Answer from the drawing. Dimensions are ordinates in mm from the lowest x, y and z of the part. A direction names the side the tool comes from. Give positions to 0.01 mm unless a question says otherwise; leave off trailing zeros. Order: outer loops, then holes, each group sorted by start corner. A loop starts at its lowest first (then second) coordinate and runs counter-clockwise, first axis right, second up. Notation, with made-up numbers: (66, 64.5) - (119, 64.5) arc R16 cw to (119, 79.5) - close; hole circle Ø1 at (89.25, -22.75). An arc over 180 degrees is marked (long way). Use a Markdown table: item, result. Add a question column.
1) Find section D-D, the plane x = 2. Determine the outline of the cut face in (y, z).
2) Flat-ended cylindrical pins translate along their axes: pin 1 (10 mm diameter, centred on x = 2.5, y = 22.5, fed in from -Z); pin 2 (10 mm diameter, centred on x = 6.5, z = 9, fed in from -Y); pin 3 (11.5 mm diameter, centred on x = 10, y = 10, fed in from -Z); pin 4 (2 mm diameter, centred on x = 10.5, y = 8.5, fed in from -Z). Find the tip coordinate at first contact, or state that the pin passes through.
3) Find section A-A, the plane y = 35. Determine the outline of the cut face in (x, z).
4) Straight lines are drawn through the part: line 1 (Y direction, x = 10, z = 2.05); line 2 (Y direction, x = 10, z = 27.1); line 3 (Z direction, x = 6.75, y = 28). For each, find the intervals that lie inside material, in ascending order.
5) The mould has two halves that part along X. Classify the marked faces 4, 5 and 6: released by +X, released by -X, zero draft, split by the parting line, or undercut.
6) Find section B-B, the plane x = 10. Determine the outline of the cut face in (y, z).
7) For the marked faces 1, 2 and 3, determine the directions among +Z, -Z, +X, -X, +Y, -Y from which every point of the face is accessible in a straight line to the end or side of a thin tool.
8) Find section C-C, the plane z = 26.5. Determine the outline of the cut face in (x, y), plus the area to 3 significant figures.
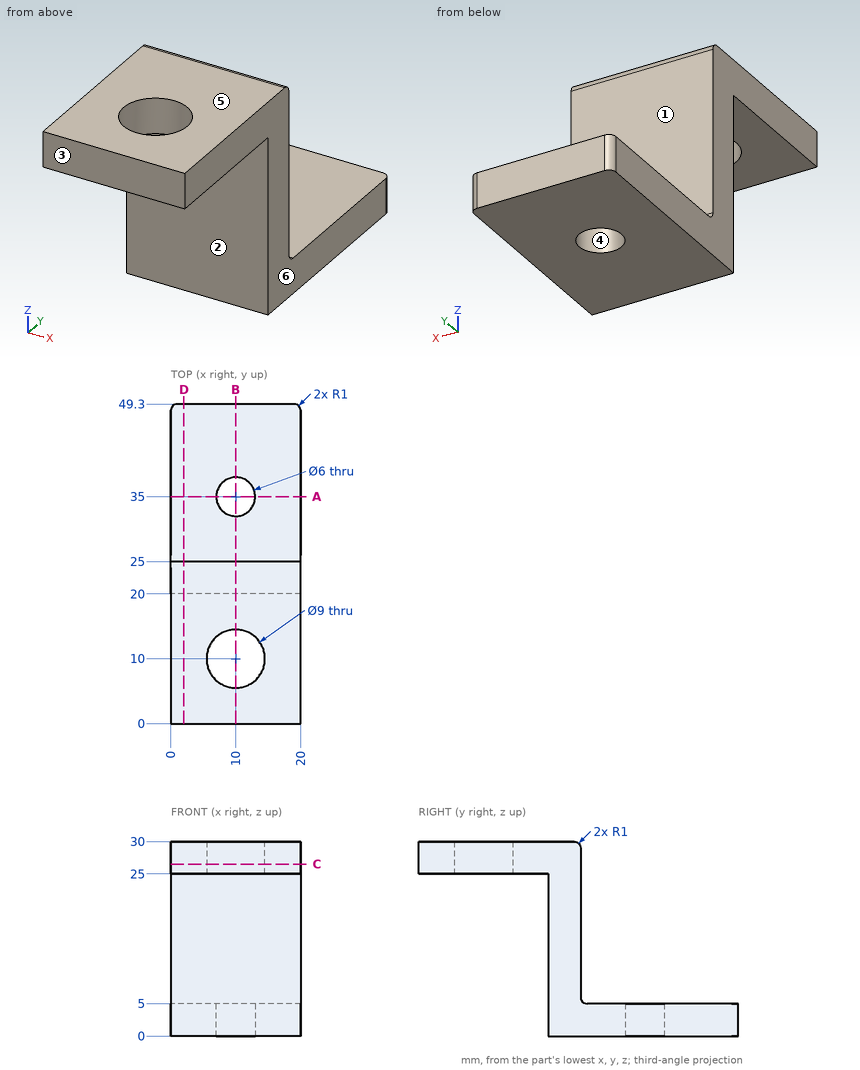
The answers:
| question | item | result |
|---|---|---|
| 1 | outline | (0, 25) - (20, 25) - (20, 0) - (49.3, 0) - (49.3, 5) - (26, 5) arc R1 cw to (25, 6) - (25, 29) arc R1 ccw to (24, 30) - (0, 30) - close |
| 2 | pin 1 | z = 0 |
| 2 | pin 2 | y = 20 |
| 2 | pin 3 | z = 25 |
| 2 | pin 4 | through |
| 3 | outline | (0, 0) - (7, 0) - (7, 5) - (0, 5) - close; (13, 0) - (20, 0) - (20, 5) - (13, 5) - close |
| 4 | line 1 | 20 to 32, 38 to 49.3 |
| 4 | line 2 | 0 to 5.5, 14.5 to 25 |
| 4 | line 3 | 0 to 5 |
| 5 | face 4 | undercut |
| 5 | face 5 | zero draft |
| 5 | face 6 | released by +X |
| 6 | outline | (0, 25) - (5.5, 25) - (5.5, 30) - (0, 30) - close; (14.5, 25) - (20, 25) - (20, 0) - (32, 0) - (32, 5) - (26, 5) arc R1 cw to (25, 6) - (25, 29) arc R1 ccw to (24, 30) - (14.5, 30) - close; (38, 0) - (49.3, 0) - (49.3, 5) - (38, 5) - close |
| 7 | face 1 | +Z, +X, -X, +Y |
| 7 | face 2 | -Z, +X, -X, -Y |
| 7 | face 3 | +Z, -Z, +X, -X, -Y |
| 8 | outline | (0, 0) - (20, 0) - (20, 25) - (0, 25) - close; hole circle Ø9 at (10, 10) |
| 8 | area | 436 mm2 |
